```python
from build123d import *

# Parameters (mm, degrees)
F2_W      = 73.1475353241
F2_H      = 70.8314999938
F0_W      = 72.4511295557
F0_H      = 71.3188424706
F5_W      = 56.9582432508
F5_H      = 55.8546073735
F6_DEPTH  = 73.152
F7_DEPTH  = 95.758
F9_DEPTH  = 86.614
F11_DEPTH = 5.08
F13_DEPTH = 1.27
F15_DEPTH = 1.524
F17_DEPTH = 0.7112


with BuildPart() as f3:
    # F2 (on offset) → F3 section 0
    with BuildSketch(Plane.XY.offset(101.6)):
        Rectangle(F2_W, F2_H)
    # F0 (on Top) → F3 section 1
    with BuildSketch(Plane.XY):
        Rectangle(F0_W, F0_H)
    loft()

    # F5 (on face) → F6 (cut)
    with BuildSketch(Plane(origin=(0, 0, 0), x_dir=(1, 0, 0), z_dir=(0, 0, -1))):
        Rectangle(F5_W, F5_H)
    extrude(amount=-F6_DEPTH, mode=Mode.SUBTRACT)

    # F4 (on face) → F7 (cut)
    with BuildSketch(Plane(origin=(-36.2251392898, 0, -0.1241505707), x_dir=(0, -1, 0), z_dir=(-0.9999941272, 0, -0.0034271736))):
        Polygon((0, 65.275169909), (-24.1607315838, -2.9297065921), (26.3105798513, -2.6568875182), align=None)
    extrude(amount=-F7_DEPTH, mode=Mode.SUBTRACT)

    # F8 (on face) → F9 (cut)
    with BuildSketch(Plane(origin=(0, 35.6592161225, 0.0855228873), x_dir=(-1, 0, 0), z_dir=(0, 0.999997124, 0.0023983321))):
        Polygon((0, 69.2265182734), (-25.3821723163, -2.8089256957), (27.3824948817, -2.8089256957), align=None)
    extrude(amount=-F9_DEPTH, mode=Mode.SUBTRACT)

    # F10 (on face) → F11 (join)
    with BuildSketch(Plane.XY.offset(101.6)):
        Polygon((-4.0646982379, 17.0300158512), (-0.5349854946, 17.0300158512), (-8.561149079, 3.1282927331), (-14.1121569056, 6.333168596), (-14.1121569056, 8.104111068), (-14.455312863, 8.104111068), (-14.455312863, 6.4796363004), (-16.1955226213, 7.6996413991), (-16.3821305686, 7.3764269532), (-14.7429471835, 6.2008514069), (-16.2762347609, 5.5274688639), (-16.0840704319, 5.0899119633), (-14.1121569056, 5.6922513065), (-8.8386744062, 2.6476047659), (-19.05, -15.0389299751), (-13.0346929654, -15.0389299751), (-11.5492390469, -15.0389299751), (11.5492390469, -15.0389299751), (13.0346929654, -15.0389299751), (19.05, -15.0389299751), (8.8386744062, 2.6476047659), (8.561149079, 3.1282927331), (0.5349854946, 17.0300158512), (4.0646982379, 17.0300158512), (4.0646982379, 18.883259967), (1.2949991506, 18.883259967), (1.2949991506, 27.9881376773), (-1.2949991506, 27.9881376773), (-1.2949991506, 18.883259967), (-4.0646982379, 18.883259967), align=None)
        Polygon((14.1121569056, 6.333168596), (8.561149079, 3.1282927331), (8.8386744062, 2.6476047659), (14.1121569056, 5.6922513065), (16.0840704319, 5.0899119633), (16.2762347609, 5.5274688639), (14.7429471835, 6.2008514069), (16.3821305686, 7.3764269532), (16.1955226213, 7.6996413991), (14.455312863, 6.4796363004), (14.455312863, 8.104111068), (14.1121569056, 8.104111068), align=None)
        Polygon((13.0346929654, -21.2668702006), (13.0346929654, -15.0389299751), (11.5492390469, -15.0389299751), (11.5492390469, -22.6051732898), (16.3196176291, -22.6051732898), (16.3196176291, -21.2668702006), align=None)
        Polygon((-11.5492390469, -15.0389299751), (-13.0346929654, -15.0389299751), (-13.0346929654, -21.2668702006), (-16.3196176291, -21.2668702006), (-16.3196176291, -22.6051732898), (-11.5492390469, -22.6051732898), align=None)
    extrude(amount=F11_DEPTH)

    # F12 (on face) → F13 (cut)
    with BuildSketch(Plane.XY.offset(106.68)):
        with BuildLine():
            add(Edge.make_bspline(
                [(0, 3.6390926689), (-9.7410636981, 3.6390926689), (-4.8705318491, -1.8195463344), (0, -7.2781853378), (4.8705318491, -1.8195463344), (9.7410636981, 3.6390926689), (0, 3.6390926689)],
                knots=[4.7123889804, 4.7123889804, 4.7123889804, 6.8067840828, 6.8067840828, 8.9011791852, 8.9011791852, 10.9955742876, 10.9955742876, 10.9955742876], degree=2, weights=[1, 0.5, 1, 0.5, 1, 0.5, 1]))
        make_face()
    extrude(amount=-F13_DEPTH, mode=Mode.SUBTRACT)

    # F14 (on face) → F15 (join)
    with BuildSketch(Plane.XY.offset(105.41)):
        with BuildLine():
            add(Edge.make_bspline(
                [(0, 2.2370060906), (-1.5068039382, 2.2370060906), (-0.7534019691, -1.1185030453), (0, -4.4740121812), (0.7534019691, -1.1185030453), (1.5068039382, 2.2370060906), (0, 2.2370060906)],
                knots=[0, 0, 0, 2.0943951024, 2.0943951024, 4.1887902048, 4.1887902048, 6.2831853072, 6.2831853072, 6.2831853072], degree=2, weights=[1, 0.5, 1, 0.5, 1, 0.5, 1]))
        make_face()
    extrude(amount=F15_DEPTH)

    # F16 (on face) → F17 (cut)
    with BuildSketch(Plane.XY.offset(106.68)):
        Polygon((2.2227161098, -7.6221204363), (0, -8.5254283622), (-2.2227161098, -7.6221204363), (-2.2227161098, -10.2890301496), (0, -9.3427076936), (2.2227161098, -10.2890301496), align=None)
    extrude(amount=-F17_DEPTH, mode=Mode.SUBTRACT)


solid = f3.part
```
Here's how the part is built. I have some questions about the finished solid (model axes, mm). A direction names the side the tool comes from. Give positions to 0.01 mm unless a question says otherwise; leave off trailing zeros. Write each question's results on one line, items separated by ' | '.
Item 1: For pin 1 Ø12 at (x, z) = (-21, 74.5) entering from +Y; pin 2 Ø1.3 at (x, y) = (0.5, -9.5) entering from +Z; pin 3 Ø10 at (x, y) = (-25, -15) entering from +Z, each with a flat end and sliding along its axis, tell me the tip position at first contact or that it passes through.
Output:
pin 1: stops at y = 35.5 | pin 2: stops at z = 106.68 | pin 3: stops at z = 101.6
Item 2: Suppose I cut it at A-A on z = 11. Give the number of separate pieces and of enclosed holes in the cut face, plus the area to 3 significant figures.
Output:
separate pieces: 4 | enclosed holes: 0 | area: 703 mm^2
Item 3: We'd pull the mould along X, two halves only. Please class faces 4 (the face through (-3, 18.883, 104)), 5 (the face through (13.035, -18, 104)), 6 (the face through (-11.3, 4.71, 104.1)): pulls with the +X half, pulls with the -X half, needs draft (parallel to the pull), parting line crosses it, or undercut.
Output:
face 4: needs draft | face 5: pulls with the +X half | face 6: undercut
Item 4: On a 3-axis mill with a long thin cutter (end or side, diameter ignored), from which of +Z, -Z, +X, -X, +Y, -Y can I reach the whole of each face in a straight line? I mean faces 1 (the face through (-15, -21.267, 104)), 2 (the face through (-1.5, 0.2, 105.41)), 3 (the face through (-11.549, -19, 104)). Say none if no direction works.
Output:
face 1: +Z, -X | face 2: +Z | face 3: +Z, -Y
Item 5: If I drill on L1, parallel to X at y = 11, z = 65.5; L2, parallel to Y at x = 30, z = 91.5; L3, parallel to Z at x = -15, y = -7, over which ranges is the centre line in solid material (lowest first)?
Output:
L1: x = -36.45 to -28.48, 28.48 to 36.45 | L2: y = -35.44 to 35.44 | L3: z = 73.15 to 101.6
